Build history of the part. All positions in model axes, mm. Coordinates: 2 decimals unless noted, no trailing zeros. Loops run counter-clockwise (first coordinate to the right, second up) from the corner with the lowest first, then second, coordinate; pieces in that order, holes last.
Item 1: Drill centre lines: line 1 along Y through (x, z) = (0, 2.45); line 2 along X through (y, z) = (116, 1.5). Where is each one in solid material? Low to high.
Item 2: Cut at A-A (y = 117). List the corners of the cut face in (x, z), and give its area (3 significant figures).
Item 3: Flat gauge pin, fed straight in: pin 1 (3 mm diameter, centred on x = 0, y = 117, fed in from -Z). Where does the tip first touch, or does it go through?
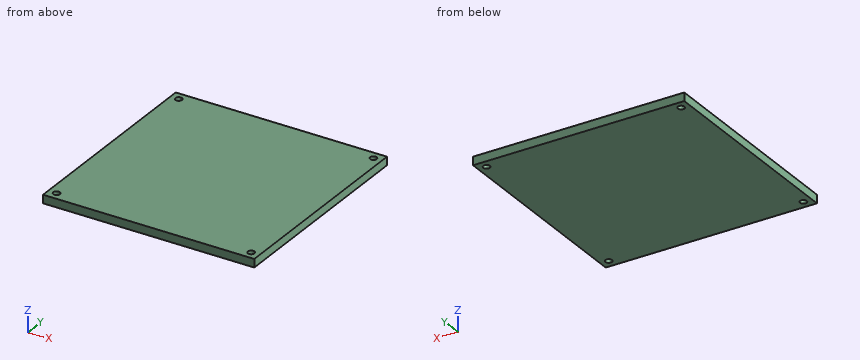
from build123d import *

# Parameters (mm, degrees)
SKETCH_2_W      = 127
SKETCH_2_H      = 127
EXTRUDE_1_DEPTH = 5


with BuildPart() as part:
    # Эскиз2 → Бобышка-Вытянуть1 (new body)
    with BuildSketch(Plane.XY):
        with Locations((58.5, 58.5)):
            Rectangle(SKETCH_2_W, SKETCH_2_H)
        with BuildLine():
            ThreePointArc((-1.981, 0), (0, -1.981), (1.981, 0))
            ThreePointArc((1.981, 0), (0, 1.981), (-1.981, 0))
        make_face(mode=Mode.SUBTRACT)
        with BuildLine():
            ThreePointArc((115.019, 0), (117, -1.981), (118.981, 0))
            ThreePointArc((118.981, 0), (117, 1.981), (115.019, 0))
        make_face(mode=Mode.SUBTRACT)
        with BuildLine():
            ThreePointArc((115.019, 117), (117, 115.019), (118.981, 117))
            ThreePointArc((118.981, 117), (117, 118.981), (115.019, 117))
        make_face(mode=Mode.SUBTRACT)
        with BuildLine():
            ThreePointArc((-1.981, 117), (0, 115.019), (1.981, 117))
            ThreePointArc((1.981, 117), (0, 118.981), (-1.981, 117))
        make_face(mode=Mode.SUBTRACT)
    extrude(amount=EXTRUDE_1_DEPTH)


solid = part.part
Filled sheet:
1. line 1: y = -5 to -1.98, 1.98 to 115.02, 118.98 to 122
1. line 2: x = -5 to -1.71, 1.71 to 115.29, 118.71 to 122
2. outline: (-5, 0) - (-1.98, 0) - (-1.98, 5) - (-5, 5) - close; (1.98, 0) - (115.02, 0) - (115.02, 5) - (1.98, 5) - close; (118.98, 0) - (122, 0) - (122, 5) - (118.98, 5) - close
2. area: 595 mm2
3. pin 1: passes through
